CAD build for the part. Positions are in the model's coordinates, mm. A direction names the side the tool comes from. Round coordinates to 2 decimals unless told otherwise and drop trailing zeros. Loops run counter-clockwise (first coordinate to the right, second up) from the corner with the lowest first, then second, coordinate; pieces in that order, holes last.
from build123d import *

# Parameters (mm, degrees)
ESQUISSE1_R                    = 2.5
BOSS_EXTRU_1_DEPTH             = 5
ESQUISSE2_W                    = 50
ESQUISSE2_H                    = 175
BOSS_EXTRU_2_DEPTH             = 5
ESQUISSE3_R                    = 2.5
BOSS_EXTRU_3_DEPTH             = 5
ESQUISSE4_W                    = 105
ESQUISSE4_H                    = 105
BOSS_EXTRU_4_DEPTH             = 3
ESQUISSE5_W                    = 105
ESQUISSE5_H                    = 105
ESQUISSE5_W_2                  = 95
ESQUISSE5_H_2                  = 95
BOSS_EXTRU_5_DEPTH             = 4
ESQUISSE6_W                    = 250
ESQUISSE6_H                    = 176
ESQUISSE6_R                    = 2.5
ESQUISSE6_R_2                  = 2.502271874
ESQUISSE6_R_3                  = 2.696378283
BOSS_EXTRU_6_DEPTH             = 5
BOSS_EXTRU_7_START             = -5
ESQUISSE8_W                    = 250
ESQUISSE8_H                    = 176
ESQUISSE8_R                    = 2.696378283
ESQUISSE8_R_2                  = 2.502271874
ESQUISSE8_R_3                  = 2.5
BOSS_EXTRU_7_DEPTH             = 5
ESQUISSE9_W                    = 8
ESQUISSE9_H                    = 144.140424184
ENL_V_MAT_EXTRU_1_DEPTH        = 296
R_P_TITION_LIN_AIRE1_COUNT     = 6
R_P_TITION_LIN_AIRE1_PITCH     = 25
R_P_TITION_LIN_AIRE1_COL_COUNT = 6
R_P_TITION_LIN_AIRE1_COL_PITCH = 25


with BuildPart() as part:
    # Esquisse1 → Boss.-Extru.1 (new body)
    with BuildSketch(Plane.XY):
        Polygon((-62.5, 88), (-62.5, -88), (62.5, -88), (62.5, 88), (25, 88), (25, 250.03), (-25, 250.03), (-25, 88), align=None)
        with Locations((-47.5, 77.5)):
            Circle(ESQUISSE1_R, mode=Mode.SUBTRACT)
        with Locations((-47.5, -10.5)):
            Circle(ESQUISSE1_R, mode=Mode.SUBTRACT)
        with Locations(Location((47.5, -10.5, 0), (0, 0, 180))):
            Circle(ESQUISSE1_R, mode=Mode.SUBTRACT)
        with Locations(Location((47.5, 77.5, 0), (0, 0, 180))):
            Circle(ESQUISSE1_R, mode=Mode.SUBTRACT)
    extrude(amount=BOSS_EXTRU_1_DEPTH)

    # Esquisse2 → Boss.-Extru.2 (add)
    with BuildSketch(Plane(origin=(0, 250.03, 0), x_dir=(1, 0, 0), z_dir=(0, 1, 0))):
        with Locations((0, 82.5)):
            Rectangle(ESQUISSE2_W, ESQUISSE2_H)
    extrude(amount=-BOSS_EXTRU_2_DEPTH)

    # Esquisse3 → Boss.-Extru.3 (add)
    with BuildSketch(Plane(origin=(0, 0, -170), x_dir=(-1, 0, 0), z_dir=(0, 0, -1))):
        Polygon((25, 88), (25, 250.03), (-25, 250.03), (-25, 88), (-62.5, 88), (-62.5, -88), (62.5, -88), (62.5, 88), align=None)
        with Locations(Location((47.5, -10.5, 0), (0, 0, 180))):
            Circle(ESQUISSE3_R, mode=Mode.SUBTRACT)
        with Locations(Location((47.5, 77.5, 0), (0, 0, 180))):
            Circle(ESQUISSE3_R, mode=Mode.SUBTRACT)
        with Locations((-47.5, 77.5)):
            Circle(ESQUISSE3_R, mode=Mode.SUBTRACT)
        with Locations((-47.5, -10.5)):
            Circle(ESQUISSE3_R, mode=Mode.SUBTRACT)
    extrude(amount=-BOSS_EXTRU_3_DEPTH)

    # Esquisse4 → Boss.-Extru.4 (add)
    with BuildSketch(Plane(origin=(0, 250.03, 0), x_dir=(1, 0, 0), z_dir=(0, 1, 0))):
        with Locations((0, 82.5)):
            Rectangle(ESQUISSE4_W, ESQUISSE4_H)
    extrude(amount=BOSS_EXTRU_4_DEPTH)

    # Esquisse5 → Boss.-Extru.5 (add)
    with BuildSketch(Plane(origin=(0, 253.03, 0), x_dir=(1, 0, 0), z_dir=(0, 1, 0))):
        with Locations((0, 82.5)):
            Rectangle(ESQUISSE5_W, ESQUISSE5_H)
        with Locations((0, 82.5)):
            Rectangle(ESQUISSE5_W_2, ESQUISSE5_H_2, mode=Mode.SUBTRACT)
    extrude(amount=BOSS_EXTRU_5_DEPTH)

    # Esquisse6 → Boss.-Extru.6 (add)
    with BuildSketch(Plane(origin=(0, 0, -170), x_dir=(-1, 0, 0), z_dir=(0, 0, -1))):
        Rectangle(ESQUISSE6_W, ESQUISSE6_H)
        with Locations((-47.5, 77.5)):
            Circle(ESQUISSE6_R, mode=Mode.SUBTRACT)
        with Locations((47.5, 77.5)):
            Circle(ESQUISSE6_R_2, mode=Mode.SUBTRACT)
        with Locations((-47.5, -10.5)):
            Circle(ESQUISSE6_R_3, mode=Mode.SUBTRACT)
        with Locations((47.5, -10.5)):
            Circle(ESQUISSE6_R_3, mode=Mode.SUBTRACT)
    extrude(amount=-BOSS_EXTRU_6_DEPTH)

    # Esquisse8 → Boss.-Extru.7 (add)
    with BuildSketch(Plane.XY.offset(5).offset(BOSS_EXTRU_7_START)):
        Rectangle(ESQUISSE8_W, ESQUISSE8_H)
        with Locations((47.5, -10.5)):
            Circle(ESQUISSE8_R, mode=Mode.SUBTRACT)
        with Locations((-47.5, 77.5)):
            Circle(ESQUISSE8_R_2, mode=Mode.SUBTRACT)
        with Locations(Location((47.5, 77.5, 0), (0, 0, 180))):
            Circle(ESQUISSE8_R_3, mode=Mode.SUBTRACT)
        with Locations((-47.5, -10.5)):
            Circle(ESQUISSE8_R, mode=Mode.SUBTRACT)
    extrude(amount=BOSS_EXTRU_7_DEPTH)

    # Esquisse9 → Enlèv. mat.-Extru.1 (cut)
    with BuildSketch(Plane(origin=(0, 0, -170), x_dir=(-1, 0, 0), z_dir=(0, 0, -1))):
        Rectangle(ESQUISSE9_W, ESQUISSE9_H)
    enl_v_mat_extru_1 = extrude(amount=-ENL_V_MAT_EXTRU_1_DEPTH, mode=Mode.SUBTRACT)

    # Répétition linéaire1: Enlèv. mat.-Extru.1 ×6
    with Locations(*[(-i * R_P_TITION_LIN_AIRE1_PITCH, 0, 0) for i in range(1, R_P_TITION_LIN_AIRE1_COUNT)]):
        add(enl_v_mat_extru_1, mode=Mode.SUBTRACT)

    # Répétition linéaire1 col: Enlèv. mat.-Extru.1 ×6
    with Locations(*[(i * R_P_TITION_LIN_AIRE1_COL_PITCH, 0, 0) for i in range(1, R_P_TITION_LIN_AIRE1_COL_COUNT)]):
        add(enl_v_mat_extru_1, mode=Mode.SUBTRACT)


solid = part.part
Item 1: Cut at A-A (y = 214.5). List the corners of the cut face in (x, z).
Verdict:
outline: (-25, -170) - (25, -170) - (25, -165) - (-25, -165) - close; (-25, 0) - (25, 0) - (25, 5) - (-25, 5) - close
Item 2: Cut at D-D (z = -108.5). List the corners of the cut face in (x, y), plus the area to 3 significant figures.
Verdict:
outline: (-52.5, 250.03) - (-25, 250.03) - (-25, 245.03) - (25, 245.03) - (25, 250.03) - (52.5, 250.03) - (52.5, 257.03) - (47.5, 257.03) - (47.5, 253.03) - (-47.5, 253.03) - (-47.5, 257.03) - (-52.5, 257.03) - close
area: 605 mm2
Item 3: Mould opens along Z. For faces 4 (the flat face through (0, 250.03, -13)), 5 (the flat face through (-1, 253, -135)), 6 (the flat face through (30, 44, -165)) say: released by +Z, released by -Z, zero draft, split by the parting line, or undercut.
Verdict:
face 4: zero draft
face 5: released by -Z
face 6: undercut
Item 4: Flat gauge pins, fed straight in: P1, Ø1.5, axis at y = 38, z = -166.5, coming from the -X side; P2, Ø4, axis at x = -74.5, z = 2, coming from the +Y side; P3, Ø1.5, axis at y = -28, z = -167, coming from the +X side. Where does each tip first touch, or does it go through?
Verdict:
P1: stops at x = -121
P2: stops at y = 88
P3: stops at x = 121
Item 5: Wall check: L1, parallel to Y at x = 47.5, z = -168.7; L2, parallel to X at y = 77, z = 2; L3, parallel to Y at x = -47, z = -166. Give the ranges that are in metal, low to high.
Verdict:
L1: y = -88 to -72.07, 72.07 to 75, 80 to 88
L2: x = -125 to -49.95, -45.05 to 45.05, 49.95 to 125
L3: y = -88 to -72.07, 72.07 to 75.05, 79.95 to 88
Item 6: 3-axis set-ups, long thin cutter, end or side, ignore diameter. For faces 1 (the flat face through (0, 245.03, -84)), 2 (the flat face through (-1, 253.03, -83)), 3 (the flat face through (0, 250.03, -153)): which of +Z, -Z, +X, -X, +Y, -Y reach the whole face in a straight line?
Verdict:
face 1: +X, -X, -Y
face 2: +Y
face 3: -Z, +X, -X, +Y
Item 7: Cut at B-B (x = 91.5). List the corners of the cut face in (y, z), plus the area to 3 significant figures.
Verdict:
outline: (-88, -170) - (88, -170) - (88, -165) - (-88, -165) - close; (-88, 0) - (88, 0) - (88, 5) - (-88, 5) - close
area: 1,760 mm2
Item 8: Cut at C-C (x = -36). List the corners of the cut face in (y, z).
Verdict:
outline: (-88, -170) - (88, -170) - (88, -165) - (-88, -165) - close; (-88, 0) - (88, 0) - (88, 5) - (-88, 5) - close; (250.03, -135) - (257.03, -135) - (257.03, -130) - (253.03, -130) - (253.03, -35) - (257.03, -35) - (257.03, -30) - (250.03, -30) - close
